```python
from build123d import *

# Parameters (mm, degrees)
BOSS_EXTRUDE1_DEPTH = 7.5
SKETCH2_W           = 3.2
SKETCH2_H           = 6
CUT_EXTRUDE1_DEPTH  = 5
FILLET1_R           = 1.5


with BuildPart() as part:
    # Sketch1 → Boss-Extrude1 (new body, symmetric)
    with BuildSketch(Plane(origin=(0, 0, 0), x_dir=(0, 0, -1), z_dir=(1, 0, 0))):
        Polygon((-1.55, 0), (-1.45, 5), (1.45, 5), (1.55, 0), (4, 0), (4, 12), (-4, 12), (-4, 0), align=None)
    extrude(amount=BOSS_EXTRUDE1_DEPTH, both=True)

    # Sketch2 → Cut-Extrude1 (cut)
    with BuildSketch(Plane(origin=(0, 12, 0), x_dir=(1, 0, 0), z_dir=(0, 1, 0))):
        Rectangle(SKETCH2_W, SKETCH2_H)
    extrude(amount=-CUT_EXTRUDE1_DEPTH, mode=Mode.SUBTRACT)

    # Fillet1
    fillet1_edges = [part.edges().sort_by_distance(p)[0] for p in [
        (1.6, 7, 0),
        (-1.6, 7, 0),
    ]]
    fillet(fillet1_edges, radius=FILLET1_R)


solid = part.part
```
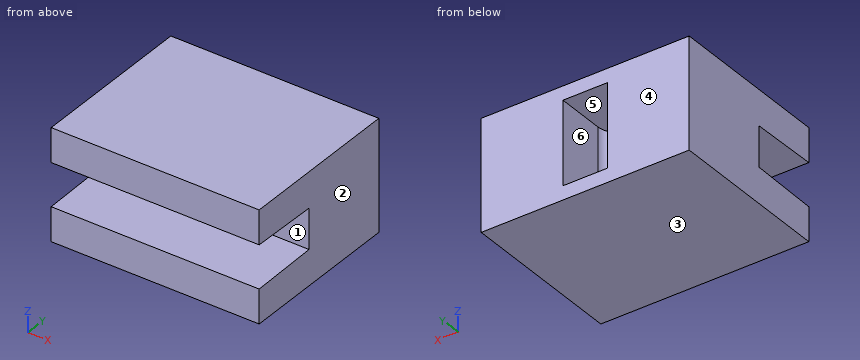
The listing builds one solid part. Answer for the finished solid, in the listing's coordinates (mm). Face numbers are marked on the shaded views. A direction names the side the tool comes from. Give positions to 0.01 mm unless a question says otherwise; leave off trailing zeros. Loops run counter-clockwise (first coordinate to the right, second up) from the corner with the lowest first, then second, coordinate; pieces in that order, holes last. Notation, with made-up numbers: (5.25, 51.5) - (28.25, 51.5) arc R19 ccw to (28.25, 70.5) - close; hole circle Ø1 at (7, 52). An arc over 180 degrees is marked (long way). Answer as CSV lines item,"result". Start each with the question number.
Item 1: A cutting plane is placed at B-B on z = 2. Determine the outline of the cut face in (x, y), then the cut area to 3 significant figures.
Item 2: The mould has two halves that part along Z. Classify the marked faces 3, 4, 5 and 6: +Z half, -Z half, draft (parallel to the pull), parting line (faces both ways), or undercut.
Item 3: Find the intervals of material crossed by line 1 (X direction, y = 10.75, z = 0.5); line 2 (Z direction, x = 1, y = 4.75) (3 decimals); line 3 (Y direction, x = 7.25, z = 1), in increasing order. Write a range as from..to.
Item 4: A cutting plane is placed at A-A on y = 4.5. Determine the outline of the cut face in (x, z), then the cut area to 3 significant figures.
Item 5: For the marked faces 1 and 2, determine the directions among +Z, -Z, +X, -X, +Y, -Y from which every point of the face is accessible in a straight line to the end or side of a thin tool.
Item 6: A cutting plane is placed at C-C on x = -6.5. Determine the outline of the cut face in (y, z), then the cut area to 3 significant figures.
Item 7: A cutting plane is placed at D-D on y = 1. Determine the outline of the cut face in (x, z).
Found:
1,outline,"(-7.5, 0) - (7.5, 0) - (7.5, 12) - (1.6, 12) - (1.6, 8.5) arc R1.5 cw to (0.1, 7) - (-0.1, 7) arc R1.5 cw to (-1.6, 8.5) - (-1.6, 12) - (-7.5, 12) - close"
1,area,"165 mm^2"
2,face 3,"-Z half"
2,face 4,"draft"
2,face 5,"undercut"
2,face 6,"undercut"
3,line 1,"x = -7.5..-1.6, 1.6..7.5"
3,line 2,"z = -4..-1.455, 1.455..4"
3,line 3,"y = 5..12"
4,outline,"(-7.5, -4) - (7.5, -4) - (7.5, -1.46) - (-7.5, -1.46) - close; (-7.5, 1.46) - (7.5, 1.46) - (7.5, 4) - (-7.5, 4) - close"
4,area,"76.2 mm^2"
5,face 1,"+X, -X, -Y"
5,face 2,"+Z, -Z, +X, +Y, -Y"
6,outline,"(0, -4) - (12, -4) - (12, 4) - (0, 4) - (0, 1.55) - (5, 1.45) - (5, -1.45) - (0, -1.55) - close"
6,area,"81.0 mm^2"
7,outline,"(-7.5, -4) - (7.5, -4) - (7.5, -1.53) - (-7.5, -1.53) - close; (-7.5, 1.53) - (7.5, 1.53) - (7.5, 4) - (-7.5, 4) - close"
